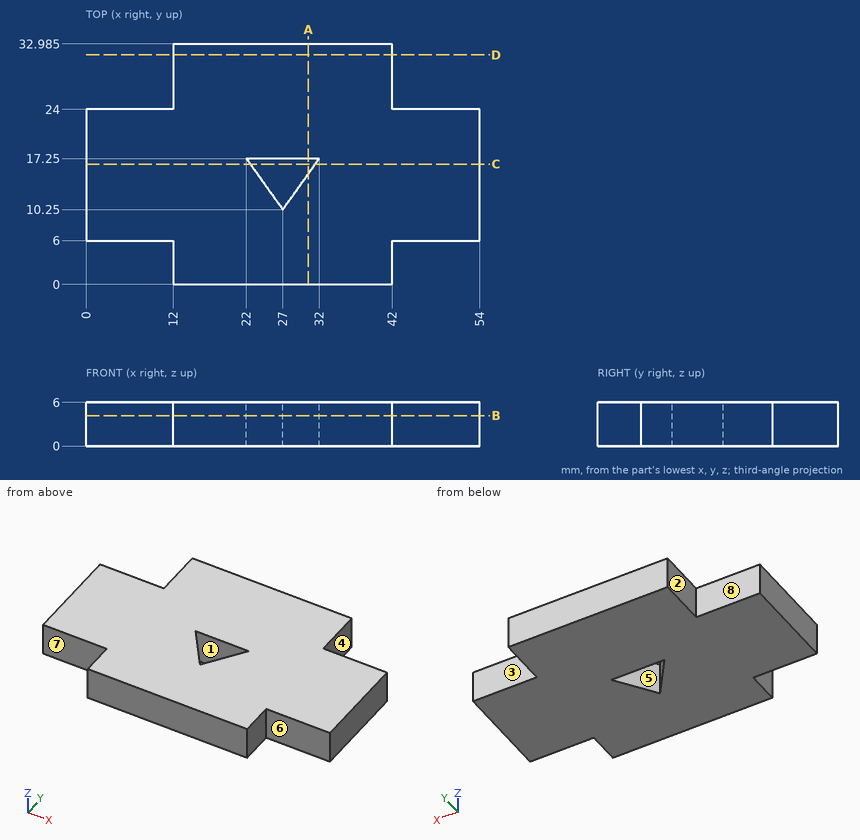
Input: dimensioned drawing with shaded views. Units: mm. Origin: part minimum x, y, z. A direction names the side the tool comes from. Coordinates: 2 decimals unless noted, no trailing zeros. Loops run counter-clockwise (first coordinate to the right, second up) from the corner with the lowest first, then second, coordinate; pieces in that order, holes last. Notation, with made-up numbers: (62.5, 55) -> (110.5, 55) arc R20 ccw to (110.5, 66) -> close; hole circle Ø8 at (61.5, -27.5). An arc over 180 degrees is marked (long way). One line per item, written item: value. Start each with the question number.
Q1. Contact query for flat-ended pins moving along their axis: P1, Ø1.5, axis at x = 43, y = 16, coming from the -Z side; P2, Ø3, axis at x = 47, z = 2, coming from the -Y side; P3, Ø3, axis at x = 7.5, z = 2, coming from the +Y side; P4, Ø1.8, axis at y = 4, z = 2.5, coming from the -X side. Output: stop coordinate, or through.
Q2. Section query C-C, the plane y = 16.5. Return the cut outline in (x, z).
Q3. Line query: line 1 along Y through (x, z) = (44, 1.05); line 2 along X through (y, z) = (10.5, 5); line 3 along X through (y, z) = (31.5, 1.9). Output: solid intervals per line, ascending.
Q4. Section query A-A, the plane x = 30.5. Return the cut outline in (y, z) (3 decimals), and give its area (3 significant figures).
Q5. Mould query, pull axis Y, two halves, no side actions, for the marked faces 1, 2 and 3. Classes: pulls with the +Y half, pulls with the -Y half, needs draft (parallel to the pull), parting line crosses it, or undercut.
Q6. Section query D-D, the plane y = 31.5. Return the cut outline in (x, z).
Q7. Section query B-B, the plane z = 4.2. Return the cut outline in (x, y) (3 decimals).
Q8. Set-up query: the marked faces 4, 5, 6, 7 and 8. Return all of +Z, -Z, +X, -X, +Y, -Y with unobstructed straight access to the full face (end or side cutting, diameter ignored); none if empty.
Results:
1. P1: z = 0
1. P2: y = 6
1. P3: y = 24
1. P4: x = 12
2. outline: (0, 0) -> (22.54, 0) -> (22.54, 6) -> (0, 6) -> close; (31.46, 0) -> (54, 0) -> (54, 6) -> (31.46, 6) -> close
3. line 1: 6 to 24
3. line 2: 0 to 26.82, 27.18 to 54
3. line 3: 12 to 42
4. outline: (0, 0) -> (15.15, 0) -> (15.15, 6) -> (0, 6) -> close; (17.25, 0) -> (32.985, 0) -> (32.985, 6) -> (17.25, 6) -> close
4. area: 185 mm^2
5. face 1: undercut
5. face 2: needs draft
5. face 3: pulls with the +Y half
6. outline: (12, 0) -> (42, 0) -> (42, 6) -> (12, 6) -> close
7. outline: (0, 6) -> (12, 6) -> (12, 0) -> (42, 0) -> (42, 6) -> (54, 6) -> (54, 24) -> (42, 24) -> (42, 32.985) -> (12, 32.985) -> (12, 24) -> (0, 24) -> close; hole (22, 17.25) -> (27, 10.25) -> (32, 17.25) -> close
8. face 4: +Z, -Z, +X, +Y
8. face 5: +Z, -Z
8. face 6: +Z, -Z, +X, -Y
8. face 7: +Z, -Z, -X, -Y
8. face 8: +Z, -Z, -X, +Y
